Can you work these out from the model? Positions are in its coordinate system, mm. Round coordinates to 2 decimals unless told otherwise and drop trailing zeros. Order: outer loops, then holes, each group sorted by start corner. A loop starts at its lowest first (then second) coordinate and runs counter-clockwise, first axis right, second up.
Q1. If we section it at A-A (y = 1.55): Please give me the cut outline in (x, z).
Q2. If I drill on line 1 (X direction, y = 4.45, z = -49.5); line 2 (Z direction, x = 32.5, y = 4.25); line 3 (X direction, y = 2.6, z = -35), over which ranges is the centre line in solid material (lowest first)?
Q3. Will these pins go through, and if not, where does the flat tip stop? P1, Ø1.5, axis at x = -119.13, z = -50.51, coming from the +Y side; P2, Ø2, axis at y = 2.5, z = -26, coming from the +X side.
Q4. If we section it at B-B (x = 68): Please give me the cut outline in (y, z), plus the area to 3 significant figures.
Q5. If we section it at C-C (z = -28): Please give me the cut outline in (x, y).
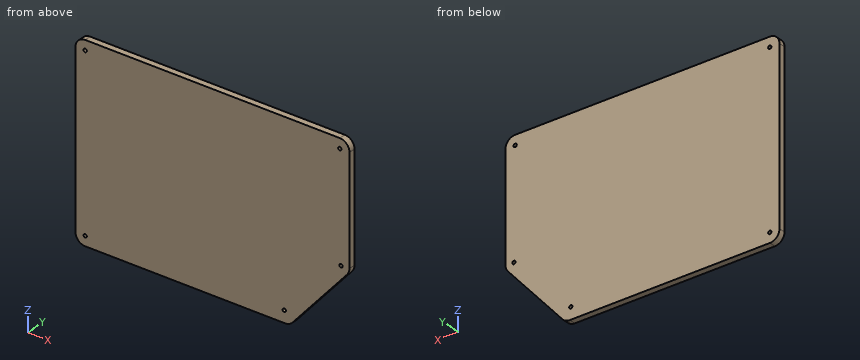
from build123d import *

# Parameters (mm, degrees)
SKETCH_2_R      = 1.25
EXTRUDE_1_DEPTH = 5


with BuildPart() as part:
    # 草图2 → 凸台-拉伸1 (new body)
    with BuildSketch(Plane(origin=(0, 0, 0), x_dir=(1, 0, 0), z_dir=(0, 1, 0))):
        with BuildLine():
            Line((-119.131169622, 57.908224798), (34.013330694, 57.908224798))
            ThreePointArc((34.013330694, 57.908224798), (37.09334763, 57.236783015), (39.614431575, 55.344304711))
            Line((39.614431575, 55.344304711), (81.469931259, 6.86767066))
            ThreePointArc((81.469931259, 6.86767066), (82.804540382, 4.611499029), (83.268830378, 2.031590747))
            Line((83.268830378, 2.031590747), (83.268830378, -79.491775202))
            ThreePointArc((83.268830378, -79.491775202), (81.101420559, -84.724365382), (75.868830378, -86.891775202))
            Line((75.868830378, -86.891775202), (-119.131169622, -86.891775202))
            ThreePointArc((-119.131169622, -86.891775202), (-124.363759802, -84.724365382), (-126.531169622, -79.491775202))
            Line((-126.531169622, -79.491775202), (-126.531169622, 50.508224798))
            ThreePointArc((-126.531169622, 50.508224798), (-124.363759802, 55.740814979), (-119.131169622, 57.908224798))
        make_face()
        with Locations(Location((76.810606689, 2.381907658, 0), (0, 0, 270))):
            Circle(SKETCH_2_R, mode=Mode.SUBTRACT)
        with Locations(Location((33.291419632, 48.931148856, 0), (0, 0, 270))):
            Circle(SKETCH_2_R, mode=Mode.SUBTRACT)
        with Locations(Location((-119.131169622, 50.508224798, 0), (0, 0, 270))):
            Circle(SKETCH_2_R, mode=Mode.SUBTRACT)
        with Locations(Location((-119.131169622, -79.491775202, 0), (0, 0, 270))):
            Circle(SKETCH_2_R, mode=Mode.SUBTRACT)
        with Locations(Location((75.868830378, -79.491775202, 0), (0, 0, 270))):
            Circle(SKETCH_2_R, mode=Mode.SUBTRACT)
    extrude(amount=EXTRUDE_1_DEPTH)


solid = part.part
Solution:
1. outline: (-126.53, -50.51) arc R7.4 ccw to (-119.13, -57.91) - (34.01, -57.91) arc R7.4 ccw to (39.61, -55.34) - (81.47, -6.87) arc R7.4 ccw to (83.27, -2.03) - (83.27, 79.49) arc R7.4 ccw to (75.87, 86.89) - (-119.13, 86.89) arc R7.4 ccw to (-126.53, 79.49) - close; hole circle Ø2.5 at (-119.13, -50.51); hole circle Ø2.5 at (-119.13, 79.49); hole circle Ø2.5 at (33.29, -48.93); hole circle Ø2.5 at (75.87, 79.49); hole circle Ø2.5 at (76.81, -2.38)
2. line 1: x = -126.53 to -119.87, -118.39 to 32.18, 34.4 to 44.66
2. line 2: z = -57.91 to -49.9, -47.96 to 86.89
2. line 3: x = -126.53 to 57.18
3. P1: passes through
3. P2: stops at x = 65.81
4. outline: (0, -22.47) - (5, -22.47) - (5, 86.89) - (0, 86.89) - close
4. area: 547 mm2
5. outline: (-126.53, 0) - (63.22, 0) - (63.22, 5) - (-126.53, 5) - close
